```python
from build123d import *

# Parameters (mm, degrees)
SKETCH_1_W          = 107.3
SKETCH_1_H          = 78.7
SKETCH_1_R          = 1.6
EXTRUDE_1_DEPTH     = 2
EXTRUDE_2_DEPTH     = 10
SKETCH_3_R          = 1.6
CUT_EXTRUDE_1_DEPTH = 11


with BuildPart() as part:
    # Эскиз1 → Бобышка-Вытянуть1 (new body)
    with BuildSketch(Plane(origin=(0, 0, 0), x_dir=(1, 0, 0), z_dir=(0, 1, 0))):
        with Locations((53.65, 39.35)):
            Rectangle(SKETCH_1_W, SKETCH_1_H)
        with Locations((3.5, 75.2)):
            Circle(SKETCH_1_R, mode=Mode.SUBTRACT)
        with Locations((96.4, 75.2)):
            Circle(SKETCH_1_R, mode=Mode.SUBTRACT)
        with Locations((96.4, 3.5)):
            Circle(SKETCH_1_R, mode=Mode.SUBTRACT)
        with Locations((3.5, 3.5)):
            Circle(SKETCH_1_R, mode=Mode.SUBTRACT)
    extrude(amount=EXTRUDE_1_DEPTH)

    # Эскиз2 → Бобышка-Вытянуть2 (add)
    with BuildSketch(Plane.XZ):
        Polygon((93.9, -4.943375673), (96.4, -6.386751346), (98.9, -4.943375673), (98.9, -2.056624327), (96.4, -0.613248654), (93.9, -2.056624327), align=None)
        Polygon((93.9, -76.643375673), (96.4, -78.086751346), (98.9, -76.643375673), (98.9, -73.756624327), (96.4, -72.313248654), (93.9, -73.756624327), align=None)
        Polygon((3.5, -6.386751346), (6, -4.943375673), (6, -2.056624327), (3.5, -0.613248654), (1, -2.056624327), (1, -4.943375673), align=None)
        Polygon((3.5, -72.313248654), (1, -73.756624327), (1, -76.643375673), (3.5, -78.086751346), (6, -76.643375673), (6, -73.756624327), align=None)
    extrude(amount=EXTRUDE_2_DEPTH)

    # Эскиз3 → Вырез-Вытянуть1 (cut, through all)
    with BuildSketch(Plane(origin=(0, 0, 0), x_dir=(1, 0, 0), z_dir=(0, 1, 0))):
        with Locations((3.5, 3.5)):
            Circle(SKETCH_3_R)
        with Locations((3.5, 75.2)):
            Circle(SKETCH_3_R)
        with Locations((96.4, 75.2)):
            Circle(SKETCH_3_R)
        with Locations((96.4, 3.5)):
            Circle(SKETCH_3_R)
    extrude(amount=-CUT_EXTRUDE_1_DEPTH, mode=Mode.SUBTRACT)


solid = part.part
```
Input: part model. Units: mm. Frame: model coordinates. A direction names the side the tool comes from. Round coordinates to 2 decimals unless told otherwise and drop trailing zeros. Write each loop counter-clockwise with the first axis right and the second up, starting at its lowest first coordinate (ties: lowest second). Pieces come first, ordered by that corner, then holes. Notation, with made-up numbers: M 46,-4 L 74,-4 A21 cw 74,35 Z; hole C 85,52.5 d1. An arc over 180 degrees is marked long. Write each question's results on one line, items separated by ' | '.
Q1. Line query: line 1 along Z through (x, y) = (96.4, 1.3); line 2 along Z through (x, y) = (96.4, -5.5); line 3 along X through (y, z) = (-4.5, -75.2). Output: solid intervals per line, ascending.
Results:
line 1: z = -78.7 to -76.8, -73.6 to -5.1, -1.9 to 0 | line 2: z = -78.09 to -76.8, -73.6 to -72.31, -6.39 to -5.1, -1.9 to -0.61 | line 3: x = 1 to 1.9, 5.1 to 6, 93.9 to 94.8, 98 to 98.9
Q2. Section query D-D (z = -29). Return loops of the section in (x, y), and give its area (3 significant figures).
Results:
outline: M 0,0 L 107.3,0 L 107.3,2 L 0,2 Z | area: 215 mm^2
Q3. Section query A-A (z = -75.2). Return loops of the section in (x, y), and give its area (3 significant figures).
Results:
outline: M 0,0 L 1,0 L 1,-10 L 1.9,-10 L 1.9,2 L 0,2 Z; M 5.1,-10 L 6,-10 L 6,0 L 93.9,0 L 93.9,-10 L 94.8,-10 L 94.8,2 L 5.1,2 Z; M 98,-10 L 98.9,-10 L 98.9,0 L 107.3,0 L 107.3,2 L 98,2 Z | area: 238 mm^2
Q4. Section query B-B (y = -3.5). Return loops of the section in (x, z).
Results:
outline: M 1,-76.64 L 3.5,-78.09 L 6,-76.64 L 6,-73.76 L 3.5,-72.31 L 1,-73.76 Z; M 1,-4.94 L 3.5,-6.39 L 6,-4.94 L 6,-2.06 L 3.5,-0.61 L 1,-2.06 Z; M 93.9,-76.64 L 96.4,-78.09 L 98.9,-76.64 L 98.9,-73.76 L 96.4,-72.31 L 93.9,-73.76 Z; M 93.9,-4.94 L 96.4,-6.39 L 98.9,-4.94 L 98.9,-2.06 L 96.4,-0.61 L 93.9,-2.06 Z; hole C 3.5,-75.2 d3.2; hole C 3.5,-3.5 d3.2; hole C 96.4,-75.2 d3.2; hole C 96.4,-3.5 d3.2
Q5. Section query C-C (x = 81). Return loops of the section in (y, z), and give its area (3 significant figures).
Results:
outline: M 0,-78.7 L 2,-78.7 L 2,0 L 0,0 Z | area: 157 mm^2
Q6. Draft query along Z for faces 1 (the face through (2.267, -4.93, -73.025)), 2 (the face through (4.732, -4.93, -77.375)), 3 (the face through (98.9, -5, -75)). Return one class per face: released by +Z, released by -Z, zero draft, split by the parting line, or undercut.
Results:
face 1: undercut | face 2: released by -Z | face 3: zero draft
Q7. Pin query (flat end, axial travel): P1, Ø1.4, axis at y = -2.5, z = -75.5, coming from the -X side; P2, Ø0.9, axis at y = -6, z = -75, coming from the +X side; P3, Ø4, axis at x = 3.5, z = -75.2, coming from the +Y side; P4, Ø10, axis at x = 24.5, z = -56.5, coming from the -Y side. Return the tip coordinate at first contact, or that it passes through.
Results:
P1: stops at x = 1 | P2: stops at x = 98.9 | P3: stops at y = 2 | P4: stops at y = 0
Q8. Access query for faces 4 (the face through (6, -5, -4)), 5 (the face through (2.233, -4.93, -77.355)), 6 (the face through (97.668, -4.93, -1.345)). Directions: +Z, -Z, +X, -X, +Y, -Y. A direction counts if a zero-diameter tool reaches every point of the face in a straight line with its end or side. Return the directions, or none.
Results:
face 4: +Z, -Z, -Y | face 5: -Z, -X, -Y | face 6: +Z, +X, -Y
